Could you check a few things on this model? Use its own coordinates, in mm. A direction names the side the tool comes from. Coordinates: 2 decimals unless noted, no trailing zeros. Write each loop counter-clockwise with the first axis right and the second up, starting at its lowest first coordinate (ties: lowest second). Pieces come first, ordered by that corner, then holes.
```python
from build123d import *

# Parameters (mm, degrees)
SKETCH2_W           = 3.175
SKETCH2_H           = 25.4
BOSS_EXTRUDE1_DEPTH = 3.175
SKETCH2_3_W         = 3.175
SKETCH2_3_H         = 25.4
BOSS_EXTRUDE2_DEPTH = 12.7


with BuildPart() as part:
    # Sketch2 → Boss-Extrude1 (new body)
    with BuildSketch(Plane.XY):
        Polygon((47.625, 0), (0, 0), (0, -19.05), (47.625, -25.4), align=None)
        with Locations((49.2125, -12.7)):
            Rectangle(SKETCH2_W, SKETCH2_H)
    extrude(amount=BOSS_EXTRUDE1_DEPTH)

    # Sketch2_3 → Boss-Extrude2 (add)
    with BuildSketch(Plane.XY):
        with Locations((49.2125, -12.7)):
            Rectangle(SKETCH2_3_W, SKETCH2_3_H)
    extrude(amount=BOSS_EXTRUDE2_DEPTH)


solid = part.part
```
1. I want a section at A-A on y = -23.25. Please give me the cut outline in (x, z) (3 decimals).
Verdict:
outline: (31.5, 0) - (50.8, 0) - (50.8, 12.7) - (47.625, 12.7) - (47.625, 3.175) - (31.5, 3.175) - close
2. I want a section at C-C on x = 10.5. Please give me the cut outline in (y, z) (3 decimals), plus the area to 3 significant figures.
Verdict:
outline: (-20.45, 0) - (0, 0) - (0, 3.175) - (-20.45, 3.175) - close
area: 64.9 mm2
3. I want a section at B-B on z = 1.5. Please give me the cut outline in (x, y) (3 decimals).
Verdict:
outline: (0, -19.05) - (47.625, -25.4) - (50.8, -25.4) - (50.8, 0) - (0, 0) - close
4. I want a section at D-D on y = -4.5. Please give me the cut outline in (x, z) (3 decimals), plus the area to 3 significant figures.
Verdict:
outline: (0, 0) - (50.8, 0) - (50.8, 12.7) - (47.625, 12.7) - (47.625, 3.175) - (0, 3.175) - close
area: 192 mm2
5. On a 3-axis mill with a long thin cutter (end or side, diameter ignored), from which of +Z, -Z, +X, -X, +Y, -Y can I reach the whole of each face in a straight line? I mean faces 1 (the face through (50.8, -13, 6)), 2 (the face through (47.625, -13, 8)). Say none if no direction works.
Verdict:
face 1: +Z, -Z, +X, +Y, -Y
face 2: +Z, -X, +Y, -Y
6. Please list where these lines run through material, in increasing order: line 1 along X through (y, z) = (-8.75, 4.5) (3 decimals); line 2 along Z through (x, y) = (41, -15.5) (3 decimals); line 3 along Y through (x, z) = (39, 1.5).
Verdict:
line 1: x = 47.625 to 50.8
line 2: z = 0 to 3.175
line 3: y = -24.25 to 0
7. For pin 1 (1 mm diameter, centred on x = 5.5, z = 1.5, fed in from -Y); pin 2 (3 mm diameter, centred on x = 37, y = -22, fed in from +Z) (3 decimals); pin 3 (2 mm diameter, centred on x = 45, z = 3, fed in from -Y), each with a flat end and sliding along its axis, tell me the tip position at first contact or that it passes through.
Verdict:
pin 1: stops at y = -19.85
pin 2: stops at z = 3.175
pin 3: stops at y = -25.18
